Verification items for the finished model (mm, model axes). Face numbers are marked on the shaded views. A direction names the side the tool comes from. Round coordinates to 2 decimals unless told otherwise and drop trailing zeros. Loops run counter-clockwise (first coordinate to the right, second up) from the corner with the lowest first, then second, coordinate; pieces in that order, holes last. Notation, with made-up numbers: (32.5, -9.75) -> (63.5, -9.75) arc R7 cw to (63.5, -5.75) -> close; hole circle Ø2 at (76.5, 47). An arc over 180 degrees is marked (long way). Write item = value, one per line.
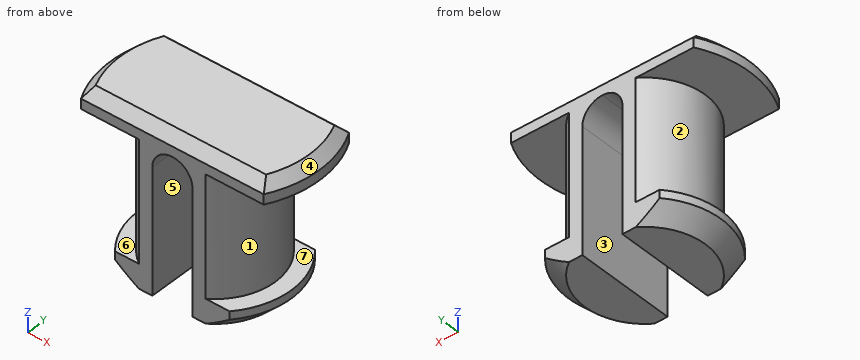
```python
from build123d import *

# Parameters (mm, degrees)
F2_W          = 32.7764776534
F2_H          = 9.1045777517
F2_W_2        = 20.9091340361
F2_H_2        = 3.5162510286
F3_DEPTH      = 25
F4_W          = 2
F4_H          = 7.2
F5_DEPTH      = 25
F5_DEPTH_BACK = 25
F6_R          = 0.99999
F7_SIZE       = 0.8
F8_SIZE       = 0.5


# Not quite as in the source:
# - a fillet or chamfer is up to 0.001 mm smaller than in the source, because OpenCascade refuses the exact size


with BuildPart() as f1:
    # F0 (on Front) → F1 (revolve)
    with BuildSketch(Plane.XZ):
        Polygon((0, 0), (0, 8.2), (-5.2, 8.2), (-5.2, 7.2), (-3, 7.2), (-3, 1.2), (-3.8, 1.2), (-3.8, 0), align=None)
    revolve(axis=Axis((0, 0, 4.1), (0, 0, 1)))

    # F2 (on Top) → F3 (cut)
    with BuildSketch(Plane.XY):
        with Locations((1.9882628694, 7.0522888758)):
            Rectangle(F2_W, F2_H)
        with Locations((1.9568684145, -4.2581255143)):
            Rectangle(F2_W_2, F2_H_2)
    extrude(amount=F3_DEPTH, mode=Mode.SUBTRACT)

    # F4 (on Front) → F5 (cut, two sides)
    with BuildSketch(Plane.XZ) as f5_sk:
        with Locations((0, 3.6)):
            Rectangle(F4_W, F4_H)
    extrude(amount=-F5_DEPTH, mode=Mode.SUBTRACT)
    extrude(f5_sk.sketch, amount=F5_DEPTH_BACK, mode=Mode.SUBTRACT)

    # F6 (radius 1 in the source; OpenCascade refuses exactly that, so slightly less here)
    f6_edges = [f1.edges().sort_by_distance(p)[0] for p in [
        (-1, 0, 7.2),
        (1, 0, 7.2),
    ]]
    fillet(f6_edges, radius=F6_R)

    # F7
    f7_edges = [f1.edges().sort_by_distance(p)[0] for p in [
        (3.8, 0, 0),
        (-3.8, 0, 0),
    ]]
    chamfer(f7_edges, length=F7_SIZE)

    # F8
    f8_edges = [f1.edges().sort_by_distance(p)[0] for p in [
        (0, -2.5, 8.2),
        (-5.2, 0, 8.2),
        (0, 2.5, 8.2),
        (5.2, 0, 8.2),
    ]]
    chamfer(f8_edges, length=F8_SIZE)


solid = f1.part
```
(1) Sectioned sample at A-A, the plane z = 1. Record the cut outline in (x, y).
Filled sheet:
outline = (-2.86, -2.5) -> (-1, -2.5) -> (-1, 2.5) -> (-2.86, 2.5) arc R3.8 ccw to start; (1, -2.5) -> (2.86, -2.5) arc R3.8 ccw to (2.86, 2.5) -> (1, 2.5) -> close
(2) Sectioned sample at D-D, the plane z = 7.5. Record the cut outline in (x, y), and give its area (3 significant figures).
Filled sheet:
outline = (-4.56, -2.5) -> (4.56, -2.5) arc R5.2 ccw to (4.56, 2.5) -> (-4.56, 2.5) arc R5.2 ccw to start
area = 49.9 mm2
(3) Draft check along Z on the marked faces 4, 5, 6 and 7. Enter one of: released by +Z, released by -Z, zero draft, split by the parting line, or undercut.
Filled sheet:
face_4 = released by +Z
face_5 = zero draft
face_6 = undercut
face_7 = undercut
(4) Go/stop test with flat-tipped pins: pin 1 Ø2 at (x, y) = (-2, 0) entering from -Z; pin 2 Ø1.5 at (y, z) = (1, 3.5) entering from -X. Record where each tip stops, or that it passes through.
Filled sheet:
pin_1 = 0
pin_2 = -2.99
(5) Material ranges on probe 1 along X at (y, z) = (0.35, 5.75); probe 2 along X at (y, z) = (-1.95, 6.5); probe 3 along Y at (x, z) = (-2.5, 3), recorded low to high. Write a range as from..to.
Filled sheet:
probe_1 = -2.98..-1, 1..2.98
probe_2 = -2.28..-0.95, 0.95..2.28
probe_3 = -1.66..1.66
(6) Set-up check for the marked faces 1, 2 and 3: record each of +Z, -Z, +X, -X, +Y, -Y from which the full face is reachable in a straight line by a thin tool's end or side.
Filled sheet:
face_1 = +X
face_2 = -X
face_3 = -Z, +Y, -Y
(7) Sectioned sample at B-B, the plane x = 4. Record the cut outline in (y, z), and give its area (3 significant figures).
Filled sheet:
outline = (-2.5, 7.2) -> (2.5, 7.2) -> (2.5, 7.7) -> (2, 8.2) -> (-2, 8.2) -> (-2.5, 7.7) -> close
area = 4.75 mm2
(8) Sectioned sample at C-C, the plane z = 3. Record the cut outline in (x, y).
Filled sheet:
outline = (-1.66, -2.5) -> (-1, -2.5) -> (-1, 2.5) -> (-1.66, 2.5) arc R3 ccw to start; (1, -2.5) -> (1.66, -2.5) arc R3 ccw to (1.66, 2.5) -> (1, 2.5) -> close
